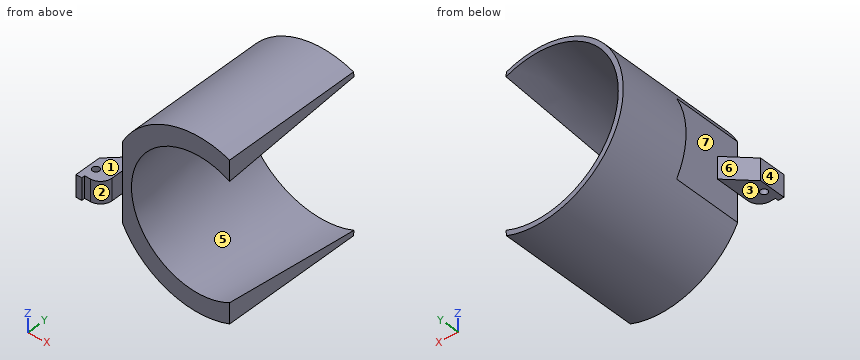
Autodesk Inventor part; units mm, degrees
ref_plane "作業平面4" through (0, 0, 37) normal (0, 0, 1) x (1, 0, 0)
ref_plane "作業平面5" through (10, -51, 41.3014) normal (0, 1, 0) x (1, 0, 0)
ref_plane "作業平面6" through (-10, -53.5, -46.9901) normal (0, 0, -1) x (-1, 0, 0)
sketch "スケッチ1" plane through (0, 0, 0) normal (0, 0, 1) x (1, 0, 0)
  line L0 (0, 0) -> (32, 0)
  line L1 (0, 0) -> (0, 30)
  line L2 (0, 30) -> (35, 30)
  line L3 (35, 30) -> (32, 0)
  line L4 (32, 0) -> (33.9901, -0.199)
  line L5 (33.9901, -0.199) -> (36.9901, 29.801)
  line L6 (36.9901, 29.801) -> (35, 30)
  line L7 (0, 0) -> (0, -80)
  line L8 (0, -80) -> (26.01, -80)
  line L9 (32, 0) -> (24.0199, -79.801)
  line L10 (33.9901, -0.199) -> (26.01, -80)
  line L11 (26.01, -80) -> (24.0199, -79.801)
  line L12 (26.01, -80) -> (36.9901, -80)
  line L13 (36.9901, -80) -> (36.9901, 29.801)
  line L14 (24.0199, -79.801) -> (24, -80)
  dimension "d0" = 32
  dimension "d1" = 30
  dimension "d2" = 35
  dimension "d3" = 2
  dimension "d4" = 80
revolve "回転1" add sketch "スケッチ1" angle 360 about axis through (0, 0, 0) along (0, 1, 0) contours L3 L6 L5 L4 | L4 L10 L11 L9 | L5 L13 L12 L10 | L11 L8 L14
ref_plane "作業平面4" through (0, 0, 37) normal (0, 0, 1) x (1, 0, 0)
sketch "スケッチ2" plane through (0, 0, 37) normal (0, 0, 1) x (1, 0, 0)
  circle A0 centre (0, 0) radius 33
  line L0 (0, 0) -> (0, -46)
  line L1 (-13.5, -41) -> (13.5, -41)
  line L2 (13.5, -41) -> (13.5, -51)
  line L3 (13.5, -51) -> (-13.5, -51)
  line L4 (-13.5, -51) -> (-13.5, -41)
  line L5 (-13.5, -41) -> (13.5, -51) construction
  line L6 (13.5, -41) -> (-13.5, -51) construction
  dimension "d10" = 66
  dimension "d11" = 46
  dimension "d12" = 27
  dimension "d13" = 10
sketch "スケッチ4" plane through (0, -80, 0) normal (0, -1, 0) x (1, 0, 0)
  circle A0 centre (0, 0) radius 36.9901
  line L0 (-20, 25.4) -> (20, 25.4)
  line L1 (20, 25.4) -> (20, -25.4)
  line L2 (20, -25.4) -> (-20, -25.4)
  line L3 (-20, -25.4) -> (-20, 25.4)
  line L4 (-20, 25.4) -> (20, -25.4) construction
  line L5 (20, 25.4) -> (-20, -25.4) construction
  arc A1 (20, 13.2808) -> (-20, 13.2808) centre (0, 0) ccw
  arc A2 (-20, -13.2808) -> (20, -13.0826) centre (-0.0647, -0.1207) ccw
  dimension "d14" = 40
  dimension "d15" = 50.8
extrude "押し出し1" add sketch "スケッチ4" along normal blind 10 contours L0 L1 A1 L3 | A2 L1 L2 L3
sketch "スケッチ5" plane through (-20, -80, 25.4) normal (0, 0, 1) x (1, 0, 0)
  line L0 (0, 0) -> (40, 0)
  line L1 (40, 0) -> (40, -10)
  line L2 (20, 0) -> (20, -5)
  line L3 (20, -5) -> (35, -5)
  line L4 (20, -5) -> (5, -5)
  circle A0 centre (5, -5) radius 1.25
  circle A1 centre (35, -5) radius 1.25
  point P0 (20, 80)
  dimension "d18" = 5
  dimension "d19" = 15
  dimension "d20" = 15
  dimension "d21" = 2.5
  dimension "d22" = 2.5
extrude "押し出し2" cut sketch "スケッチ5" against normal blind 51
extrude "押し出し3" cut sketch "スケッチ2" against normal blind 80 contours L1 L2 L3 L4
sketch "スケッチ6" plane through (0, -80, 0) normal (0, -1, 0) x (1, 0, 0)
  arc A0 (-20, -13.2808) -> (2.6513, -23.8531) centre (-0.0647, -0.1207) ccw
  arc A1 (20, -13.2665) -> (2.6513, -23.8531) centre (0, 0) ccw
  line L0 (20, -13.2665) -> (20, -25.4)
  line L1 (-20, -25.4) -> (-20, -13.2808)
  line L2 (20, 25.4) -> (20, 13.2808)
  arc A2 (20, 13.2808) -> (-20, 13.2808) centre (0, 0) ccw
  line L3 (-20, 13.2808) -> (-20, 25.4)
  arc A3 (-20, 13.2808) -> (-20, -13.2808) centre (0.1181, 0) ccw
  arc A4 (-20, 25.4) -> (-20, -25.4) centre (1.0675, 0) ccw
  arc A5 (20, -13.2665) -> (20, 13.2808) centre (0.0108, 0.0072) ccw
  arc A6 (20, -25.4) -> (20, 25.4) centre (-1.0675, 0) ccw
  dimension "d27" = 33
  dimension "d28" = 33
extrude "押し出し4" add sketch "スケッチ6" along normal blind 10 contours L1 A4 L3 A3 A1 | A5 L2 A6 L0
sketch "スケッチ7" plane through (0, -51, 0) normal (0, 1, 0) x (1, 0, 0)
  arc A0 (13.5, 34.4386) -> (-13.5, 34.4386) centre (0, 0) ccw
  line L0 (-10, 26.9901) -> (10, 26.9901)
  line L1 (10, 26.9901) -> (10, 46.9901)
  line L2 (10, 46.9901) -> (-10, 46.9901)
  line L3 (-10, 46.9901) -> (-10, 26.9901)
  line L4 (-10, 26.9901) -> (10, 46.9901) construction
  line L5 (10, 26.9901) -> (-10, 46.9901) construction
  point P0 (0, 36.9901)
  dimension "d31" = 20
extrude "押し出し5" add sketch "スケッチ7" against normal blind 5
mirror "ミラー1" about plane through (0, 0, 0) normal (0, 0, 1) of "押し出し5"
ref_plane "作業平面5" through (10, -51, 41.3014) normal (0, 1, 0) x (1, 0, 0)
sketch "スケッチ8" plane through (10, -51, 41.3014) normal (0, 1, 0) x (1, 0, 0)
  line L0 (-14.9767, 1.255) -> (-4.9767, 1.255)
  line L1 (-4.9767, 1.255) -> (-4.9767, 81.255)
  line L2 (-4.9767, 81.255) -> (-14.9767, 81.255)
  line L3 (-14.9767, 81.255) -> (-14.9767, 1.255)
  line L4 (-14.9767, 1.255) -> (-4.9767, 81.255) construction
  line L5 (-4.9767, 1.255) -> (-14.9767, 81.255) construction
  line L6 (-9.9767, 81.255) -> (-9.9767, 1.255)
  circle A0 centre (-9.9767, 81.255) radius 1
  circle A1 centre (-9.9767, 1.255) radius 1
  point P0 (-9.9767, 41.255)
  dimension "d42" = 10
  dimension "d43" = 80
  dimension "d44" = 2
  dimension "d45" = 2
extrude "押し出し7" cut sketch "スケッチ8" against normal blind 5 contours L6 A1 L0 | L0 A1 | L0 A1 L6 | A0 L2 L6 | L6 L2 A0 | L2 A0
ref_plane "作業平面6" through (-10, -53.5, -46.9901) normal (0, 0, -1) x (-1, 0, 0)
sketch "スケッチ9" plane through (-10, -53.5, -46.9901) normal (0, 0, -1) x (-1, 0, 0)
  line L0 (26.829, -26.5556) -> (-47.1085, -26.5556)
  line L1 (-0.028, -26.5556) -> (-0.028, 22.4444)
  line L2 (-23.7626, 22.4444) -> (28.9336, 22.4444)
  line L3 (28.9336, 22.4444) -> (28.9336, 86.0653)
  line L4 (28.9336, 86.0653) -> (-23.7626, 86.0653)
  line L5 (-23.7626, 86.0653) -> (-23.7626, 22.4444)
  line L6 (-23.7626, 86.0653) -> (-48.5643, 86.0653)
  line L7 (-48.5643, 86.0653) -> (-48.5643, -39.6917)
  line L8 (-48.5643, -39.6917) -> (-23.7626, -39.6917)
  line L9 (-23.7626, -39.6917) -> (-23.7626, 86.0653)
  line L10 (-23.7626, 22.4444) -> (28.9336, 22.4444)
  line L11 (28.9336, 22.4444) -> (28.9336, -39.6917)
  line L12 (28.9336, -39.6917) -> (-23.7626, -39.6917)
  line L13 (-23.7626, -39.6917) -> (-23.7626, 22.4444)
  point P0 (-10, 53.5)
  dimension "d48" = 49
extrude "押し出し9" cut sketch "スケッチ9" against normal blind 95 contours L1 L2 L11 L12 L9 L0 | L0 L9 L2 L1 | L9 L8 L7 L6 L5
sketch "スケッチ10" plane through (0, -31.0556, 0) normal (0, -1, 0) x (1, 0, 0)
  arc A0 (13.7626, 34.3345) -> (13.7626, -34.3345) centre (0, 0) ccw
  arc A1 (13.7626, 25.4063) -> (13.7626, -25.4063) centre (0, 0) ccw
  line L0 (13.7626, 25.4063) -> (13.7626, 34.3345)
  line L1 (-28.8944, 0) -> (-32.8944, 0)
  line L2 (-32.8944, 0) -> (-32.8944, 16.9181)
  line L3 (-32.8944, 0) -> (-32.8944, -16.9181)
  dimension "d53" = 4
extrude "押し出し10" cut sketch "スケッチ10" against normal blind 30 contours L2 L3 A0
sketch "スケッチ11" plane through (-32.8944, -31.0556, -16.9181) normal (-1, 0, 0) x (0, 0, 1)
  line L0 (33.8361, 0) -> (0, 0)
  line L1 (0, 0) -> (0, 30)
  line L2 (16.9181, 0) -> (16.9181, 5)
  line L3 (12.1681, 10) -> (21.6681, 10)
  line L4 (21.6681, 10) -> (21.6681, 0)
  line L5 (21.6681, 0) -> (12.1681, 0)
  line L6 (12.1681, 0) -> (12.1681, 10)
  line L7 (12.1681, 10) -> (21.6681, 0) construction
  line L8 (21.6681, 10) -> (12.1681, 0) construction
  point P0 (16.9181, 31.0556)
  dimension "d56" = 5
  dimension "d57" = 9.5
extrude "押し出し11" add sketch "スケッチ11" along normal blind 10
sketch "スケッチ12" plane through (0, -31.0556, 0) normal (0, -1, 0) x (1, 0, 0)
  line L0 (-42.8944, 4.75) -> (-32.8944, 4.75)
  line L1 (-32.8944, 4.75) -> (-32.8944, -4.75)
  line L2 (-32.8944, -4.75) -> (-42.8944, -4.75)
  line L3 (-42.8944, -4.75) -> (-42.8944, 4.75)
  line L4 (-42.8944, 4.75) -> (-32.8944, -4.75) construction
  line L5 (-32.8944, 4.75) -> (-42.8944, -4.75) construction
  point P0 (-37.8944, 0)
extrude "押し出し12" add sketch "スケッチ12" along normal blind 10
sketch "スケッチ13" plane through (-42.8944, -21.0556, 4.75) normal (0, 0, 1) x (1, 0, 0)
  line L0 (0, 0) -> (0, -20)
  line L1 (0, -20) -> (0, -15)
  line L2 (0, -15) -> (3, -15)
  circle A0 centre (3, -15) radius 1.5
  point P0 (42.8944, 21.0556)
  dimension "d62" = 3
  dimension "d63" = 3
extrude "押し出し13" cut sketch "スケッチ13" against normal blind 10
chamfer "面取り1" distance 10 angle 45 1 edges at (-42.8944, -21.0556, 0)
fillet "フィレット2" radius 5 1 edges at (-32.8944, -41.0556, 0)
sketch "スケッチ14" plane through (0, -41.0556, 0) normal (0, -1, 0) x (1, 0, 0)
  line L0 (-42.8944, -4.75) -> (-37.8944, -4.75)
  line L1 (-42.8944, 4.75) -> (-40.3944, 4.75)
  line L2 (-40.3944, 4.75) -> (-40.3944, -4.75)
  line L3 (-40.3944, -4.75) -> (-42.8944, -4.75)
  line L4 (-42.8944, -4.75) -> (-42.8944, 4.75)
  point P0 (0, 0)
extrude "押し出し14" add sketch "スケッチ14" along normal blind 1.4
properties part number "知能ロボコン吸引部２.1.2"
Read the model definition and answer for the solid it produces. Units are mm, in the model's axes. Face numbers are marked on the shaded views. A direction names the side the tool comes from. Coordinates: 2 decimals unless noted, no trailing zeros. Order: outer loops, then holes, each group sorted by start corner. A loop starts at its lowest first (then second) coordinate and runs counter-clockwise, first axis right, second up. Notation, with made-up numbers: M 23,39 L 74,39 A27 cw 74,72 Z; hole C -34,81 d10. An arc over 180 degrees is marked long. Put each result on its own line as item: value. Start each with the question number.
Item 1: Consider probe 1 along Z at (x, y) = (-16, 16.5); probe 2 along Z at (x, y) = (-8, -23); probe 3 along X at (y, z) = (22, -28.5). Determine where each line is inside the solid, lowest interval first. Write a range as [from, to].
Item 2: Section A-A, the plane x = 0 is taken. Determine the outline of the cut face in (y, z), plus the area to 3 significant figures.
Item 3: For the marked faces 1, 2 and 3, determine the directions among +Z, -Z, +X, -X, +Y, -Y from which every point of the face is accessible in a straight line to the end or side of a thin tool.
Item 4: Section B-B, the plane y = -25 is taken. Determine the outline of the cut face in (x, z), plus the area to 3 significant figures.
Item 5: The mould has two halves that part along Y. Classify the marked faces 4, 5, 6 and 7: +Y half, -Y half, draft (parallel to the pull), parting line (faces both ways), or undercut.
Item 6: Section D-D, the plane y = -9 is taken. Determine the outline of the cut face in (x, z).
Item 7: Given pin 1 Ø1 at (x, y) = (-1.5, 14) entering from -Z; pin 2 Ø5 at (x, y) = (-32, -24.5) entering from +Z; pin 3 Ø4 at (y, z) = (-3, -20.5) entering from +X, each flat-ended and moving along its own axis, determine where each tip first touches the part or whether it passes through.
Computed:
1. probe 1: z = [-33.35, -29.6], [29.6, 33.35]
1. probe 2: z = [-36.11, -28.6], [28.6, 36.11]
1. probe 3: x = [-23.58, -18.9]
2. outline: M -31.06,-36.99 L 29.8,-36.99 L 30,-35 L -31.06,-28.89 Z; M -31.06,28.89 L 30,35 L 29.8,36.99 L -31.06,36.99 Z
2. area: 615 mm2
3. face 1: +Z, -X, -Y
3. face 2: +Z, -Z, +X, -Y
3. face 3: -Z, -X, -Y
4. outline: M -36.84,-4.75 L -32.89,-4.75 L -32.89,-16.92 A36.99 ccw 13.76,-34.33 L 13.76,-26.09 A29.5 cw long 13.76,26.09 L 13.76,34.33 A36.99 ccw -32.89,16.92 L -32.89,4.75 L -36.84,4.75 Z
4. area: 939 mm2
5. face 4: draft
5. face 5: +Y half
5. face 6: undercut
5. face 7: undercut
6. outline: M -32.89,-16.92 A36.99 ccw 13.76,-34.33 L 13.76,-27.89 A31.1 cw long 13.76,27.89 L 13.76,34.33 A36.99 ccw -32.89,16.92 Z
7. pin 1: stops at z = -36.98
7. pin 2: stops at z = 22.32
7. pin 3: stops at x = -22.31
